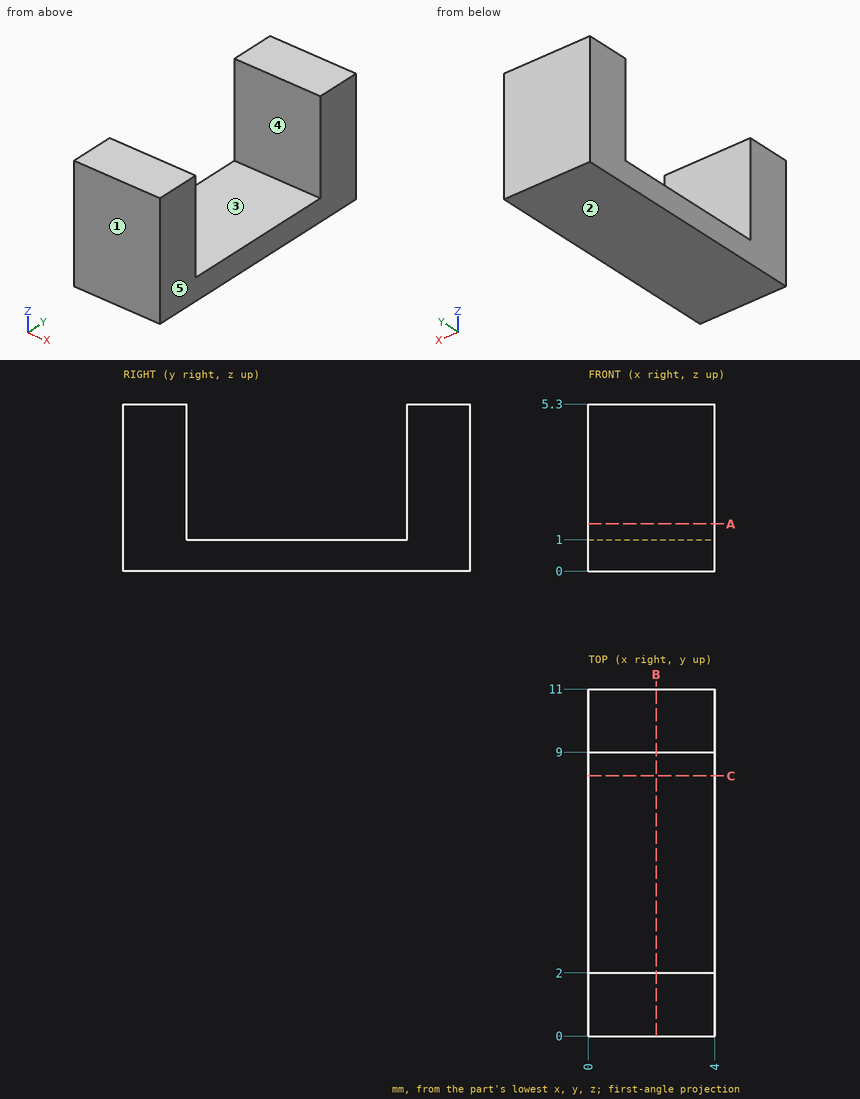
Drawing for the job (mm, zero at the part's lowest x, y, z). A direction names the side the tool comes from. Round coordinates to 2 decimals unless told otherwise and drop trailing zeros. Write each loop counter-clockwise with the first axis right and the second up, starting at its lowest first coordinate (ties: lowest second). Pieces come first, ordered by that corner, then holes. Notation, with made-up numbers: M -15.75,-19 L 43.25,-19 A34 cw 43.25,14 Z; hole C 22.5,87 d4. An arc over 180 degrees is marked long. Put each result on its own line as item: value.
Item 1: Cut at C-C (y = 8.25). List the corners of the cut face in (x, z).
Responses:
outline: M 0,0 L 4,0 L 4,1 L 0,1 Z
Item 2: Probe L1, parallel to Y at x = 0.2, z = 3.8; L2, parallel to Z at x = 2.05, y = 5. List the from-to ranges inside material, lowest first. Write a range as from..to.
Responses:
L1: 0..2, 9..11
L2: 0..1
Item 3: Cut at B-B (x = 2.15). List the corners of the cut face in (y, z), and give its area (3 significant figures).
Responses:
outline: M 0,0 L 11,0 L 11,5.3 L 9,5.3 L 9,1 L 2,1 L 2,5.3 L 0,5.3 Z
area: 28.2 mm²
Item 4: Cut at A-A (z = 1.5). List the corners of the cut face in (x, y), and give its area (3 significant figures).
Responses:
outline: M 0,0 L 4,0 L 4,2 L 0,2 Z; M 0,9 L 4,9 L 4,11 L 0,11 Z
area: 16.0 mm²
Item 5: Tool access for the marked faces 4 and 5: list every direction of +Z, -Z, +X, -X, +Y, -Y with a clear straight run to the whole face (end or side of a thin tool).
Responses:
face 4: +Z, +X, -X
face 5: +Z, -Z, +X, +Y, -Y
Item 6: Mould opens along Y. For the marked faces 1, 2 and 3 say: +Y half, -Y half, draft (parallel to the pull), parting line (faces both ways), or undercut.
Responses:
face 1: -Y half
face 2: draft
face 3: undercut
